Check sheet for the modelled part. Datum: model origin and axes. Units: mm. A direction names the side the tool comes from. Give positions to 0.01 mm unless a question says otherwise; leave off trailing zeros. Loops run counter-clockwise (first coordinate to the right, second up) from the corner with the lowest first, then second, coordinate; pieces in that order, holes last. Notation, with made-up numbers: (-1.5, 84) - (46.5, 84) arc R17 ccw to (46.5, 91) - close; hole circle Ø5 at (-23, 73.25). An arc over 180 degrees is marked (long way). Use one line per item in the form item = value.
from build123d import *

# Parameters (mm, degrees)
F0_R          = 11.938
F2_DEPTH      = 1.524
F3_DEPTH      = 2.54
F3_DEPTH_BACK = 25.4
F4_R          = 8.89
F5_DEPTH      = 1.524
F6_R          = 8.89
F7_DEPTH      = 1.524
F8_R          = 0.635
F9_DEPTH      = 25.4
F9_DEPTH_BACK = 25.4


with BuildPart() as f2:
    # F0 (on Top) → F2 (new body)
    with BuildSketch(Plane.XY):
        Circle(F0_R)
    extrude(amount=F2_DEPTH)

    # F1 (on face) → F3 (cut, two sides)
    with BuildSketch(Plane.XY) as f3_sk:
        with BuildLine():
            Line((-9.492772, 7.239), (9.492772, 7.239))
            ThreePointArc((9.492772, 7.239), (0, 11.938), (-9.492772, 7.239))
        make_face()
        with BuildLine():
            Line((9.492772, -7.239), (-9.492772, -7.239))
            ThreePointArc((-9.492772, -7.239), (0, -11.938), (9.492772, -7.239))
        make_face()
    extrude(amount=F3_DEPTH, mode=Mode.SUBTRACT)
    extrude(f3_sk.sketch, amount=-F3_DEPTH_BACK, mode=Mode.SUBTRACT)

    # F4 (on face) → F5 (join)
    with BuildSketch(Plane(origin=(0, 0, 0), x_dir=(1, 0, 0), z_dir=(0, 0, -1))):
        Circle(F4_R)
    extrude(amount=-F5_DEPTH)

    # F6 (on face) → F7 (join)
    with BuildSketch(Plane(origin=(0, 0, 0), x_dir=(1, 0, 0), z_dir=(0, 0, -1))):
        Circle(F6_R)
    extrude(amount=F7_DEPTH)

    # F8 (on face) → F9 (cut, two sides)
    with BuildSketch(Plane.XY.offset(1.524)) as f9_sk:
        Circle(F8_R)
    extrude(amount=-F9_DEPTH, mode=Mode.SUBTRACT)
    extrude(f9_sk.sketch, amount=-F9_DEPTH_BACK, mode=Mode.SUBTRACT)


solid = f2.part
Item 1: Thickness scan on L1, parallel to Y at x = 0, z = -0.2 (3 decimals); L2, parallel to Z at x = 8.75, y = -3.25; L3, parallel to Y at x = 6.5, z = 1.15. Record the ranges inside material, lowest first.
Answer block:
L1 = -8.89 to -0.635, 0.635 to 8.89
L2 = 0 to 1.52
L3 = -7.24 to 7.24
Item 2: Access from +Z, -Z, +X, -X, +Y, -Y to the whole of each face (thin tool, end or side, straight path). Record for faces 1 (the face through (-7, -7.239, 1)), 2 (the face through (-9.3, 0.1, 0)), 3 (the face through (8.48, -2.67, -0.32)).
Answer block:
face_1 = +Z, -Z, -X, -Y
face_2 = -Z, -X
face_3 = -Z
Item 3: Section check C-C on z = 1.05. Record the boundary of the cut face in (x, y) (3 decimals), then the cut area to 3 significant figures.
Answer block:
outline = (-9.493, -7.239) - (-5.16, -7.239) arc R8.89 ccw to (5.16, -7.239) - (9.493, -7.239) arc R11.938 ccw to (9.493, 7.239) - (5.16, 7.239) arc R8.89 ccw to (-5.16, 7.239) - (-9.493, 7.239) arc R11.938 ccw to start; hole circle Ø1.27 at (0, 0)
area = 345 mm2
Item 4: Section check D-D on y = 3.5. Record the boundary of the cut face in (x, z), then the cut area to 3 significant figures.
Answer block:
outline = (-11.41, 0) - (-8.17, 0) - (-8.17, -1.52) - (8.17, -1.52) - (8.17, 0) - (11.41, 0) - (11.41, 1.52) - (-11.41, 1.52) - close
area = 59.7 mm2
Item 5: Gauge pin test, flat ends, axial feed: P1, Ø0.8, axis at x = 7.5, z = 0.5, coming from the +Y side; P2, Ø0.8, axis at x = -6.5, z = 0.5, coming from the -Y side; P3, Ø1.5, axis at x = 0, y = 0, coming from the +Z side. Record the tip position at first contact, or that the pin passes through.
Answer block:
P1 = 7.24
P2 = -7.24
P3 = 1.52
Item 6: Section check A-A on x = 0. Record the boundary of the cut face in (y, z) (3 decimals), then the cut area to 3 significant figures.
Answer block:
outline = (-8.89, -1.524) - (-0.635, -1.524) - (-0.635, 1.524) - (-8.89, 1.524) - close; (0.635, -1.524) - (8.89, -1.524) - (8.89, 1.524) - (0.635, 1.524) - close
area = 50.3 mm2
Item 7: Section check B-B on y = 0. Record the boundary of the cut face in (x, z) (3 decimals).
Answer block:
outline = (-11.938, 0) - (-8.89, 0) - (-8.89, -1.524) - (-0.635, -1.524) - (-0.635, 1.524) - (-11.938, 1.524) - close; (0.635, -1.524) - (8.89, -1.524) - (8.89, 0) - (11.938, 0) - (11.938, 1.524) - (0.635, 1.524) - close
